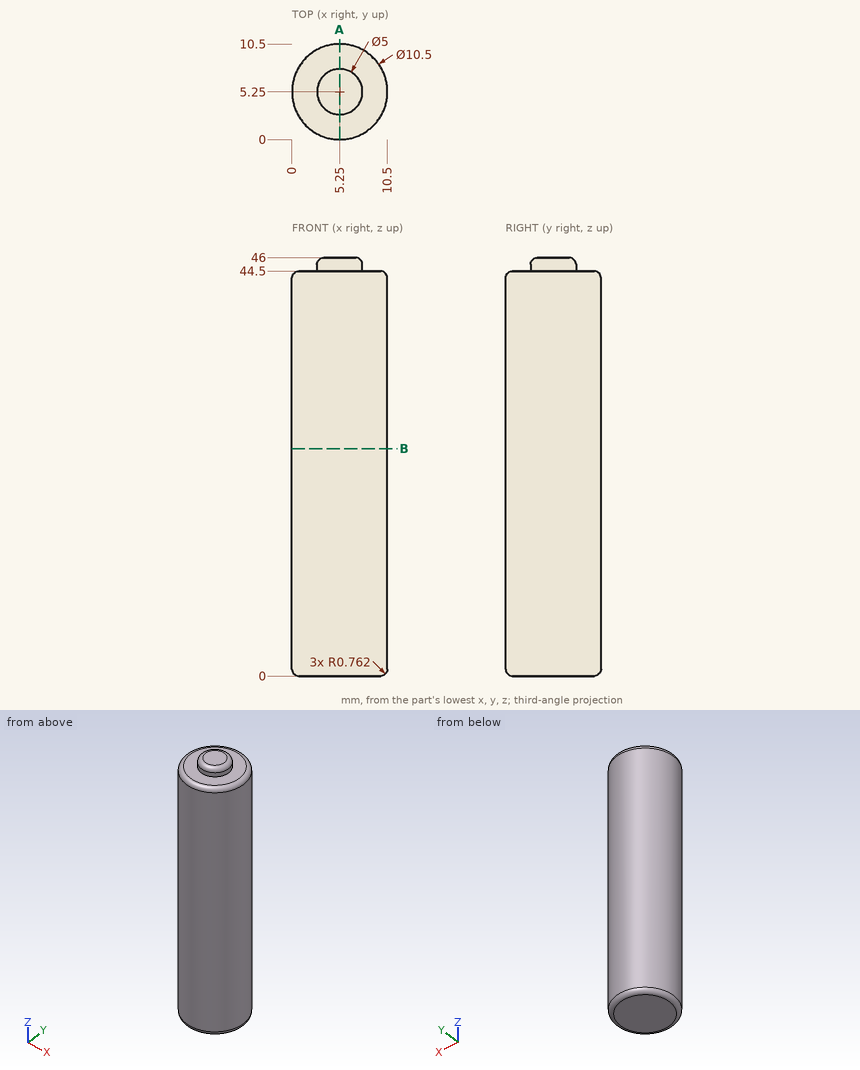
Check sheet for the drawn part. Datum: minimum x, y, z corner. Units: mm. Round coordinates to 2 decimals unless told otherwise and drop trailing zeros. Loops run counter-clockwise (first coordinate to the right, second up) from the corner with the lowest first, then second, coordinate; pieces in that order, holes last. Notation, with made-up numbers: M 35,-4.75 L 42,-4.75 A6 cw 42,-0.75 Z; hole C -6.75,47.25 d8. An arc over 180 degrees is marked long. One line per question, with ' | ' between items. Start each with the question number.
Item 1: Section check A-A (x = 5.25). Record the boundary of the cut face in (y, z), and give its area (3 significant figures).
Item 2: Section check B-B (z = 25). Record the boundary of the cut face in (x, y).
Item 3: Gauge pin test, flat ends, axial feed: pin 1 Ø3 at (x, z) = (7, 29.5) entering from -Y; pin 2 Ø1.5 at (x, y) = (2.5, 5) entering from +Z; pin 3 Ø1 at (y, z) = (6, 18.5) entering from +X. Record the tip position at first contact, or that the pin passes through.
Item 4: Scan lines: probe 1 along X at (y, z) = (5, 3); probe 2 along Z at (x, y) = (4.75, 2.5). Record each from-to range of solid material in increasing order.
Worked out:
1) outline: M 0,0.76 A0.76 ccw 0.76,0 L 9.74,0 A0.76 ccw 10.5,0.76 L 10.5,43.74 A0.76 ccw 9.74,44.5 L 7.75,44.5 L 7.75,45.24 A0.76 ccw 6.99,46 L 3.51,46 A0.76 ccw 2.75,45.24 L 2.75,44.5 L 0.76,44.5 A0.76 ccw 0,43.74 Z | area: 474 mm^2
2) outline: C 5.25,5.25 d10.5
3) pin 1: y = 0.01 | pin 2: z = 45.95 | pin 3: x = 10.49
4) probe 1: 0.01 to 10.49 | probe 2: 0 to 44.5
